The figure shows three views and two pictorial views of one solid part (mm, origin at its lowest corner). Answer the questions. Give positions to 0.01 mm unless a question says otherwise; leave off trailing zeros. Write each loop counter-clockwise with the first axis right and the second up, starting at its lowest first coordinate (ties: lowest second). Pieces come first, ordered by that corner, then holes. Notation, with made-up numbers: (27.25, 30) - (31.25, 30) arc R25 cw to (31.25, 43) - close; hole circle Ø5 at (-21.75, 16.25). An arc over 180 degrees is marked (long way). One line per question, with ' | ' between items. Start each with the question number.
1. A cutting plane is placed at A-A (x = 14). Determine the outline of the cut face in (y, z), then the cut area to 3 significant figures.
2. A cutting plane is placed at D-D (z = 14). Determine the outline of the cut face in (x, y).
3. Find the intervals of material crossed by L1, parallel to X at y = 0.8, z = 27; L2, parallel to Z at x = 14, y = 0.55; L3, parallel to Z at x = 15.5, y = 2.95, in increasing order. Write a range as from..to.
4. A cutting plane is placed at B-B (z = 27). Determine the outline of the cut face in (x, y), then the cut area to 3 significant figures.
5. A cutting plane is placed at C-C (y = 1.6). Determine the outline of the cut face in (x, z).
6. Given P1, Ø1.6, axis at y = 2, z = 22, coming from the -X side; P2, Ø10, axis at x = 13, z = 25.5, coming from the +Y side; P3, Ø1.5, axis at x = 3, y = 2.5, coming from the -Z side, each flat-ended and moving along its own axis, determine where each tip first touches the part or whether it passes through.
7. The mould has two halves that part along X. Classify the marked faces 1 and 2: +X half, -X half, draft (parallel to the pull), parting line (faces both ways), or undercut.
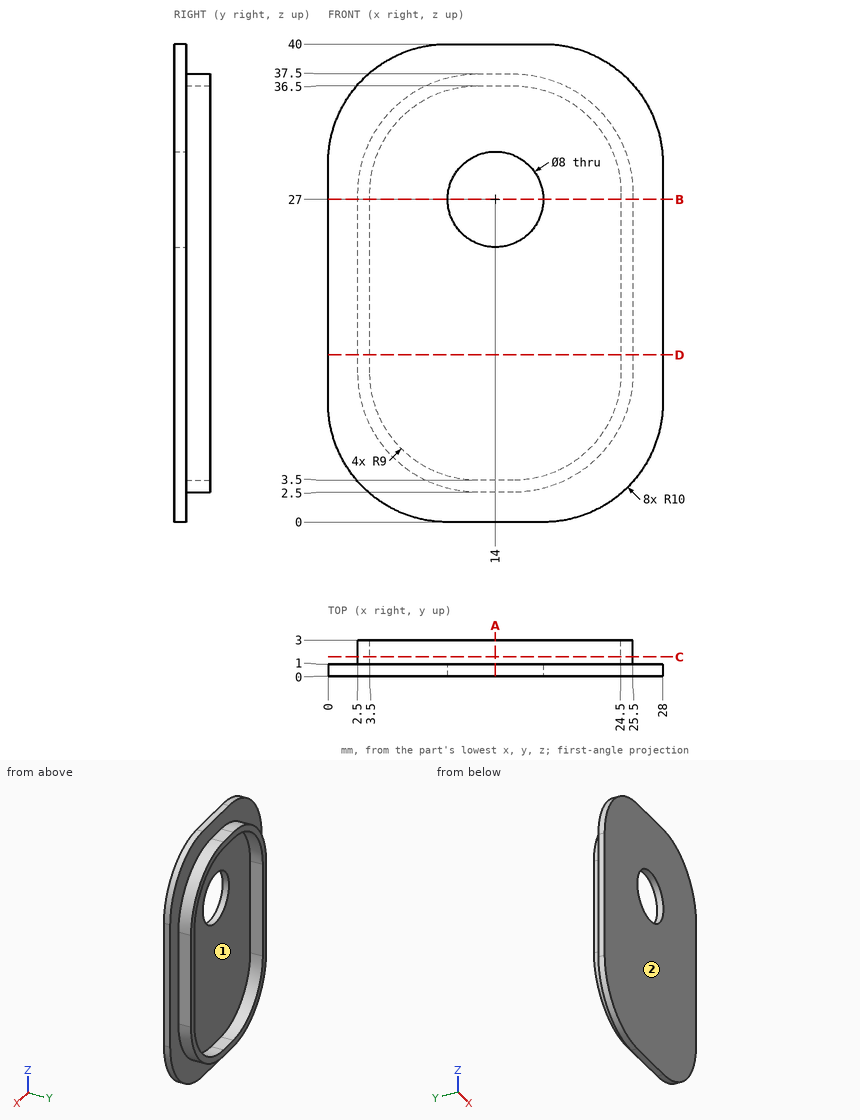
Determined:
1) outline: (0, 0) - (1, 0) - (1, 2.5) - (3, 2.5) - (3, 3.5) - (1, 3.5) - (1, 23) - (0, 23) - close; (0, 31) - (1, 31) - (1, 36.5) - (3, 36.5) - (3, 37.5) - (1, 37.5) - (1, 40) - (0, 40) - close | area: 36.0 mm2
2) outline: (0, 0) - (28, 0) - (28, 1) - (25.5, 1) - (25.5, 3) - (24.5, 3) - (24.5, 1) - (3.5, 1) - (3.5, 3) - (2.5, 3) - (2.5, 1) - (0, 1) - close
3) L1: 0..10, 18..28 | L2: 0..23, 31..40 | L3: 2.5..3.5, 36.5..37.5
4) outline: (0, 0) - (10, 0) - (10, 1) - (3.5, 1) - (3.5, 3) - (2.5, 3) - (2.5, 1) - (0, 1) - close; (18, 0) - (28, 0) - (28, 1) - (25.5, 1) - (25.5, 3) - (24.5, 3) - (24.5, 1) - (18, 1) - close | area: 24.0 mm2
5) outline: (2.5, 12.5) arc R10 ccw to (12.5, 2.5) - (15.5, 2.5) arc R10 ccw to (25.5, 12.5) - (25.5, 27.5) arc R10 ccw to (15.5, 37.5) - (12.5, 37.5) arc R10 ccw to (2.5, 27.5) - close; hole (3.5, 12.5) arc R9 ccw to (12.5, 3.5) - (15.5, 3.5) arc R9 ccw to (24.5, 12.5) - (24.5, 27.5) arc R9 ccw to (15.5, 36.5) - (12.5, 36.5) arc R9 ccw to (3.5, 27.5) - close
6) P1: x = 2.5 | P2: y = 1 | P3: z = 7.66
7) face 1: undercut | face 2: draft
